```python
from build123d import *

# Parameters (mm, degrees)
SKETCH1_R           = 36.5
BOSS_EXTRUDE1_DEPTH = 100
SKETCH2_R           = 31
CUT_EXTRUDE2_DEPTH  = 101
CUT_EXTRUDE4_DEPTH  = 101


with BuildPart() as part:
    # Sketch1 → Boss-Extrude1 (new body)
    with BuildSketch(Plane(origin=(0, 0, 0), x_dir=(1, 0, 0), z_dir=(0, 1, 0))):
        Circle(SKETCH1_R)
    extrude(amount=BOSS_EXTRUDE1_DEPTH)

    # Sketch2 → Cut-Extrude2 (cut, through all)
    with BuildSketch(Plane(origin=(0, 0, 0), x_dir=(1, 0, 0), z_dir=(0, 1, 0))):
        Circle(SKETCH2_R)
    extrude(amount=CUT_EXTRUDE2_DEPTH, mode=Mode.SUBTRACT)

    # Sketch4 → Cut-Extrude4 (cut, through all)
    with BuildSketch(Plane(origin=(0, 0, 0), x_dir=(1, 0, 0), z_dir=(0, 1, 0))):
        with BuildLine():
            Line((36.5, 0), (-36.5, 0))
            ThreePointArc((-36.5, 0), (0, -36.5), (36.5, 0))
        make_face()
    extrude(amount=CUT_EXTRUDE4_DEPTH, mode=Mode.SUBTRACT)


solid = part.part
```
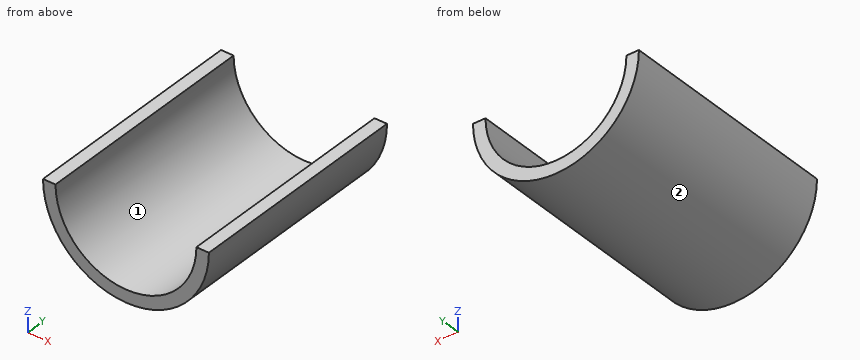
The model under review builds one solid part; all positions refer to its coordinate system, in mm. Face numbers are marked on the shaded views. Round coordinates to 2 decimals unless told otherwise and drop trailing zeros. Loops run counter-clockwise (first coordinate to the right, second up) from the corner with the lowest first, then second, coordinate; pieces in that order, holes last.
1) Consider section C-C on z = -27. State the section outline as (x, y) points.
Values follow:
outline: (-24.56, 0) - (-15.23, 0) - (-15.23, 100) - (-24.56, 100) - close; (15.23, 0) - (24.56, 0) - (24.56, 100) - (15.23, 100) - close
2) Clearance check with flat-ended pins moving along their axes: P1, Ø5, axis at x = 21.5, y = 20.5, coming from the +Z side; P2, Ø3, axis at x = 21, y = 67, coming from the +Z side; P3, Ø2, axis at y = 88, z = -14, coming from the -X side. State where each tip first meets the part, or that it passes through.
Values follow:
P1: stops at z = -19.62
P2: stops at z = -21.32
P3: stops at x = -34.11
3) Consider section A-A on z = -17.5. State the section outline as (x, y) points, then the cut area to 3 significant figures.
Values follow:
outline: (-32.03, 0) - (-25.59, 0) - (-25.59, 100) - (-32.03, 100) - close; (25.59, 0) - (32.03, 0) - (32.03, 100) - (25.59, 100) - close
area: 1,290 mm2
4) Consider section B-B on y = 14.5. State the section outline as (x, z) points.
Values follow:
outline: (-36.5, 0) arc R36.5 ccw to (36.5, 0) - (31, 0) arc R31 cw to (-31, 0) - close
5) Wall thickness on line 1 along X through (y, z) = (76.5, -5); line 2 along X through (y, z) = (60, -33); line 3 along X through (y, z) = (5, -24.5): over which ranges is each line inside the solid? List them lowest first.
Values follow:
line 1: x = -36.16 to -30.59, 30.59 to 36.16
line 2: x = -15.6 to 15.6
line 3: x = -27.06 to -18.99, 18.99 to 27.06
6) The part is to be moulded in two halves that separate along X. For the marked faces 1 and 2, say which applies: pulls with the +X half, pulls with the -X half, needs draft (parallel to the pull), parting line crosses it, or undercut.
Values follow:
face 1: undercut
face 2: parting line crosses it
7) Consider section D-D on x = 12. State the section outline as (y, z) points.
Values follow:
outline: (0, -34.47) - (100, -34.47) - (100, -28.58) - (0, -28.58) - close
